Check sheet for the modelled part. Datum: model origin and axes. Units: mm. Face numbers are marked on the shaded views. A direction names the side the tool comes from. Round coordinates to 2 decimals unless told otherwise and drop trailing zeros. Order: outer loops, then holes, each group sorted by start corner. A loop starts at its lowest first (then second) coordinate and runs counter-clockwise, first axis right, second up.
Q1. Cross-section at A-A on z = 13.25. Record the cut outline in (x, y), then the cut area to 3 significant figures.
Q2. Scan lines: probe 1 along Y at (x, z) = (-24, 15.5); probe 2 along X at (y, z) = (-6, 7.5); probe 3 along Z at (x, y) = (-18, -1). Record each from-to range of solid material in increasing order.
Q3. Cross-section at D-D on y = -12.5. Record the cut outline in (x, z), then the cut area to 3 significant figures.
Q4. Cross-section at C-C on x = -20.5. Record the cut outline in (y, z).
Q5. Cross-section at B-B on x = -9. Record the cut outline in (y, z).
Q6. Depth check by flat-ended pin: P1, Ø7.5, axis at x = 35.88, y = -13.56, coming from the +Z side; P2, Ø9.5, axis at y = -11, z = 13, coming from the -X side; P3, Ø1.9, axis at y = -27.5, z = 7.5, coming from the +X side; P4, Ø2, axis at x = 30.5, z = 13.5, coming from the -Y side. Enter the tip coordinate at first touch or a pass-through.
Q7. Set-up check for the marked faces 1, 2, 3, 4 and 5: record each of +Z, -Z, +X, -X, +Y, -Y from which the full face is reachable in a straight line by a thin tool's end or side.
Q8. Mould release check, pull along Y, two halves, no side actions. Record for the marked faces 6, 7, 8 and 9: +Y half, -Y half, draft (parallel to the pull), parting line (faces both ways), or undercut.
from build123d import *

# Parameters (mm, degrees)
F1_DEPTH = 19.05
F3_D     = 12.7
F5_D     = 12.7


with BuildPart() as f1:
    # F0 (on Top) → F1 (new body)
    with BuildSketch(Plane.XY):
        Polygon((45.4040161939, -4.0381300203), (-1.6949172365, -4.0381300203), (-1.6949172365, 2.3118699797), (-27.0949172365, 2.3118699797), (-27.0949172365, -4.0381300203), (-7.1481281937, -4.0381300203), (-7.1481281937, -23.0881300203), (-27.0949172365, -23.0881300203), (-27.0949172365, -29.4381300203), (-1.6949172365, -29.4381300203), (-1.6949172365, -23.0881300203), (45.4040161939, -23.0881300203), align=None)
    extrude(amount=F1_DEPTH)

    # F3 (through all)
    with Locations(Plane.XZ.offset(29.4381300203)):
        with Locations((-17.5699172365, 9.525)):
            Hole(F3_D / 2)

    # F5 (through all)
    with Locations(Plane(origin=(0, 0, 0), x_dir=(1, 0, 0), z_dir=(0, 0, -1))):
        with Locations((35.8790161939, 13.5631300203)):
            Hole(F5_D / 2)


solid = f1.part
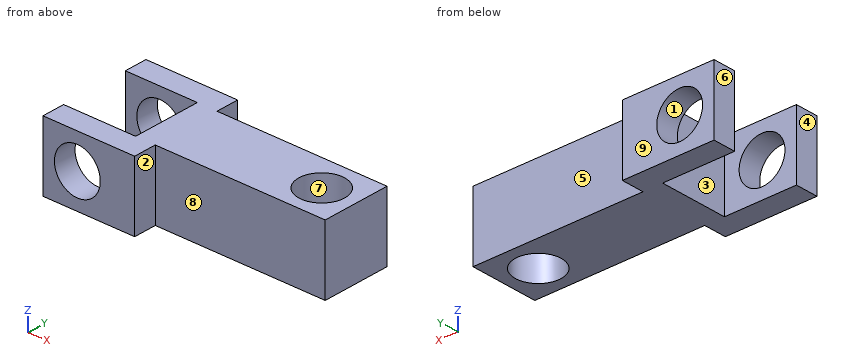
Results found:
1. outline: (-27.09, -29.44) - (-22.71, -29.44) - (-22.71, -23.09) - (-27.09, -23.09) - close; (-27.09, -4.04) - (-22.71, -4.04) - (-22.71, 2.31) - (-27.09, 2.31) - close; (-12.43, -29.44) - (-1.69, -29.44) - (-1.69, -23.09) - (45.4, -23.09) - (45.4, -4.04) - (-1.69, -4.04) - (-1.69, 2.31) - (-12.43, 2.31) - (-12.43, -4.04) - (-7.15, -4.04) - (-7.15, -23.09) - (-12.43, -23.09) - close; hole circle Ø12.7 at (35.88, -13.56)
1. area: 1,070 mm2
2. probe 1: y = -29.44 to -23.09, -4.04 to 2.31
2. probe 2: x = -7.15 to 45.4
2. probe 3: z = 0 to 3.19, 15.86 to 19.05
3. outline: (-7.15, 0) - (29.62, 0) - (29.62, 19.05) - (-7.15, 19.05) - close; (42.14, 0) - (45.4, 0) - (45.4, 19.05) - (42.14, 19.05) - close
3. area: 763 mm2
4. outline: (-29.44, 0) - (-23.09, 0) - (-23.09, 3.89) - (-29.44, 3.89) - close; (-29.44, 15.16) - (-23.09, 15.16) - (-23.09, 19.05) - (-29.44, 19.05) - close; (-4.04, 0) - (2.31, 0) - (2.31, 3.89) - (-4.04, 3.89) - close; (-4.04, 15.16) - (2.31, 15.16) - (2.31, 19.05) - (-4.04, 19.05) - close
5. outline: (-29.44, 0) - (-23.09, 0) - (-23.09, 19.05) - (-29.44, 19.05) - close; (-4.04, 0) - (2.31, 0) - (2.31, 19.05) - (-4.04, 19.05) - close
6. P1: passes through
6. P2: stops at x = -7.15
6. P3: stops at x = -1.69
6. P4: stops at y = -23.09
7. face 1: +Y, -Y
7. face 2: +Z, -Z, +X, -Y
7. face 3: +Z, -Z, -X
7. face 4: +Z, -Z, -X, +Y, -Y
7. face 5: +Z, -Z, +X, +Y
8. face 6: draft
8. face 7: undercut
8. face 8: -Y half
8. face 9: +Y half
